The model under review builds one solid part; all positions refer to its coordinate system, in mm. Round coordinates to 2 decimals unless told otherwise and drop trailing zeros. Loops run counter-clockwise (first coordinate to the right, second up) from the corner with the lowest first, then second, coordinate; pieces in that order, holes last. Notation, with made-up numbers: M 88,42 L 126,42 A19 ccw 126,77 Z; hole C 33.25,-2.5 d4. An arc over 180 degrees is marked long. Answer as a JSON object with one key per item and string values. Group by question number.
Item 1: Consider section B-B (x = -5.5). Give the boundary of the cut face in (y, z).
Item 2: Consider section D-D (z = 35). Give the boundary of the cut face in (x, y).
Item 3: Consider section A-A (z = -197). Give the boundary of the cut face in (x, y).
Item 4: Consider section C-C (y = -27). Give the boundary of the cut face in (x, z), and give its area (3 significant figures).
Item 5: To check wall thickness, follow line 1 (X direction, y = 0, z = 8); line 2 (X direction, y = 32, z = -97). State the ranges of each line that lie inside material, in increasing order.
Item 6: Insertion check: P1, Ø12, axis at x = -31.5, z = -155, coming from the -Y side; P2, Ø1.5, axis at y = -11.5, z = 118.5, coming from the -X side; P3, Ø5, axis at y = -9, z = 106.5, coming from the -X side; P4, Ø6, axis at y = -0.5, z = -25, coming from the +X side. Each pin has a flat end and moves straight along its axis. Give the tip position at first contact, or say it passes through.
```python
from build123d import *

# Parameters (mm, degrees)
SKETCH1_R           = 39.2557
SKETCH1_R_2         = 38.1
BOSS_EXTRUDE1_DEPTH = 228.6
SKETCH3_W           = 3.175
SKETCH3_H           = 127
CUT_EXTRUDE1_DEPTH  = 236.24451102
CIRPATTERN1_COUNT   = 4


with BuildPart() as part:
    # Sketch1 → Boss-Extrude1 (new, symmetric)
    with BuildSketch(Plane.XY):
        Circle(SKETCH1_R)
        Circle(SKETCH1_R_2, mode=Mode.SUBTRACT)
    extrude(amount=BOSS_EXTRUDE1_DEPTH, both=True)

    # Sketch3 → Cut-Extrude1 (cut, through all)
    with BuildSketch(Plane(origin=(0, 0, 0), x_dir=(1, 0, 0), z_dir=(0, 1, 0))):
        with Locations((0, 146.05)):
            Rectangle(SKETCH3_W, SKETCH3_H)
    cut_extrude1 = extrude(amount=CUT_EXTRUDE1_DEPTH, mode=Mode.SUBTRACT)

    # CirPattern1: Cut-Extrude1 ×4 about axis
    cirpattern1_axis = Axis((0, 0, 0), (0, 0, 1))
    for i in range(1, CIRPATTERN1_COUNT):
        add(cut_extrude1.rotate(cirpattern1_axis, i * 360 / CIRPATTERN1_COUNT), mode=Mode.SUBTRACT)


solid = part.part
```
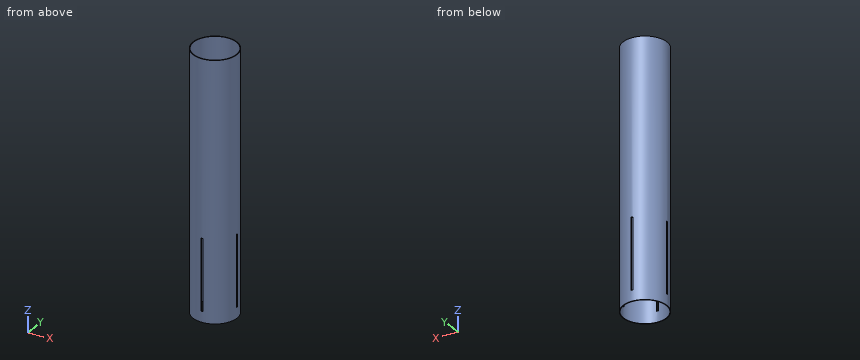
Geometry results:
{
 "1": {"outline": "M -38.87,-228.6 L -37.7,-228.6 L -37.7,228.6 L -38.87,228.6 Z; M 37.7,-228.6 L 38.87,-228.6 L 38.87,228.6 L 37.7,228.6 Z"},
 "2": {"outline": "C 0,0 d78.51; hole C 0,0 d76.2"},
 "3": {"outline": "M -39.22,-1.59 A39.26 ccw -1.59,-39.22 L -1.59,-38.07 A38.1 cw -38.07,-1.59 Z; M -39.22,1.59 L -38.07,1.59 A38.1 cw -1.59,38.07 L -1.59,39.22 A39.26 ccw Z; M 1.59,-39.22 A39.26 ccw 39.22,-1.59 L 38.07,-1.59 A38.1 cw 1.59,-38.07 Z; M 1.59,38.07 A38.1 cw 38.07,1.59 L 39.22,1.59 A39.26 ccw 1.59,39.22 Z"},
 "4": {"outline": "M -28.5,-228.6 L -26.88,-228.6 L -26.88,228.6 L -28.5,228.6 Z; M 26.88,-228.6 L 28.5,-228.6 L 28.5,228.6 L 26.88,228.6 Z", "area": "1,480 mm^2"},
 "5": {"line 1": "x = -39.26 to -38.1, 38.1 to 39.26", "line 2": "x = -22.74 to -20.68, 20.68 to 22.74"},
 "6": {"P1": "stops at y = -29.85", "P2": "stops at x = -37.76", "P3": "stops at x = -38.71", "P4": "stops at x = 39.26"}
}
